```python
from build123d import *

# Parameters (mm, degrees)
BOSS_EXTRUDE2_DEPTH = 20
SHELL1_START        = 3
SHELL1_DEPTH        = 17


# Read off the part's stored shape, not the designer's step: Shell1
with BuildPart() as part:
    # Sketch1 → Boss-Extrude2 (new body)
    with BuildSketch(Plane(origin=(0, 0, 0), x_dir=(1, 0, 0), z_dir=(0, 1, 0))):
        Polygon((111.6, 38.05), (28, 53.55), (0, 53.55), (0, -158.05), (26, -158.05), (63, -88.05), (111.6, -38.05), (119.1, -30.55), (119.1, 30.55), align=None)
        Polygon((84.62, 3.05), (84.62, 8.02), (49.98, 8.02), (49.98, -8.02), (84.62, -8.02), (84.62, -3.05), (88.2, -3.05), (88.2, -30.55), (111.6, -30.55), (111.6, 30.55), (88.2, 30.55), (88.2, 3.05), align=None, mode=Mode.SUBTRACT)
    extrude(amount=BOSS_EXTRUDE2_DEPTH)

    # Shell1 outline → Shell1 (cut)
    with BuildSketch(Plane(origin=(0, 0, 0), x_dir=(1, 0, 0), z_dir=(0, 1, 0)).offset(SHELL1_START)):
        Polygon((114.6, -30.807359313), (116.1, -29.307359313), (116.1, 29.307359313), (114.6, 30.807359313), align=None)
        Polygon((109.463620332, -35.943738981), (111.857359313, -33.55), (85.2, -33.55), (85.2, -11.02), (46.98, -11.02), (46.98, 11.02), (85.2, 11.02), (85.2, 33.55), (111.857359313, 33.55), (110.13729107, 35.270068243), (27.724239787, 50.55), (3, 50.55), (3, -155.05), (24.192413563, -155.05), (60.548822095, -86.26760548), align=None)
    extrude(amount=SHELL1_DEPTH, mode=Mode.SUBTRACT)


solid = part.part
```
The model under review builds one solid part; all positions refer to its coordinate system, in mm. A direction names the side the tool comes from. Round coordinates to 2 decimals unless told otherwise and drop trailing zeros. Write each loop counter-clockwise with the first axis right and the second up, starting at its lowest first coordinate (ties: lowest second). Pieces come first, ordered by that corner, then holes.
(1) We need section B-B on z = 103. Give the boundary of the cut face in (x, y), and give its area (3 significant figures).
(2) We need section A-A on x = 53. Give the boundary of the cut face in (y, z), and give its area (3 significant figures).
(3) We need section C-C on x = 69. Give the boundary of the cut face in (y, z).
(4) Mouldability with a two-part tool opening along Z and no side actions: class faces 1 (the flat face through (111.6, 10, 0)), 2 (the flat face through (86, 20, 20)), 3 (the flat face through (13, 10, 158.05)), 4 (the flat face through (84.66, 11.38, 61.46)) as +Z half, -Z half, draft (parallel to the pull), parting line (faces both ways), or undercut.
(5) Insertion check: pin 1 (5 mm diameter, centred on y = 10.5, z = -1.5, fed in from -X); pin 2 (1.5 mm diameter, centred on x = 31.5, y = 17.5, fed in from -Z); pin 3 (10 mm diameter, centred on x = 73, y = 8.5, fed in from +Z); pin 4 (6 mm diameter, centred on x = 65.5, y = 14, fed in from -Z). Each pin has a flat end and moves straight along its axis. Give the tip position at first contact, or say it passes through.
(6) Machinability: for faces 5 (the flat face through (46.98, 11, 0)), 6 (the flat face through (0, 10, 51)), 7 (the flat face through (68, 10, -8.02)), which of the approach directions +Z, -Z, +X, -X, +Y, -Y give a long, thin tool a straight path to every point of the face, cutting with its end or side? Answer none if there is none.
(7) Wall thickness on L1, parallel to X at y = 12, z = -15; L2, parallel to X at y = 17, z = -7; L3, parallel to Z at x = 89.5, y = 12: over which ranges is each line inside the solid? List them lowest first.
(8) We need section D-D on y = 16. Give the number of separate pieces and of enclosed holes in the cut face, and give its area (3 significant figures).
Findings below:
1. outline: (0, 0) - (55.1, 0) - (55.1, 20) - (51.7, 20) - (51.7, 3) - (3, 3) - (3, 20) - (0, 20) - close
1. area: 274 mm2
2. outline: (0, -48.91) - (20, -48.91) - (20, -45.86) - (3, -45.86) - (3, -11.02) - (20, -11.02) - (20, -8.02) - (0, -8.02) - close; (0, 8.02) - (20, 8.02) - (20, 11.02) - (3, 11.02) - (3, 100.55) - (20, 100.55) - (20, 106.97) - (0, 106.97) - close
2. area: 683 mm2
3. outline: (0, -45.95) - (20, -45.95) - (20, -42.9) - (3, -42.9) - (3, -11.02) - (20, -11.02) - (20, -8.02) - (0, -8.02) - close; (0, 8.02) - (20, 8.02) - (20, 11.02) - (3, 11.02) - (3, 77.57) - (20, 77.57) - (20, 81.88) - (0, 81.88) - close
4. face 1: undercut
4. face 2: draft
4. face 3: +Z half
4. face 4: undercut
5. pin 1: stops at x = 0
5. pin 2: stops at z = -53.04
5. pin 3: stops at z = 82.91
5. pin 4: stops at z = -47.15
6. face 5: +Y
6. face 6: +Z, -Z, -X, +Y, -Y
6. face 7: +Y, -Y
7. L1: x = 0 to 3, 85.2 to 88.2, 111.6 to 114.6, 116.1 to 119.1
7. L2: x = 0 to 3, 46.98 to 49.98, 84.62 to 88.2, 111.6 to 114.6, 116.1 to 119.1
7. L3: z = -42.15 to -39.1, -33.55 to -30.55, 30.55 to 33.55, 56.48 to 60.79
8. separate pieces: 1
8. enclosed holes: 3
8. area: 2,510 mm2
